Check sheet for the modelled part. Datum: model origin and axes. Units: mm. A direction names the side the tool comes from. Round coordinates to 2 decimals unless told otherwise and drop trailing zeros. Order: outer loops, then holes, each group sorted by start corner. A loop starts at its lowest first (then second) coordinate and runs counter-clockwise, first axis right, second up. Notation, with made-up numbers: (-38.75, 50) -> (-3.75, 50) arc R24 cw to (-3.75, 89) -> close; hole circle Ø2 at (27.5, 30.5). An arc over 180 degrees is marked (long way). Answer in a Markdown table with one row per item. Add a question column.
1. Depth check by flat-ended pin: P1, Ø10, axis at y = 105, z = 904.5, coming from the +X side; P2, Ø3, axis at x = 2, z = 1144.5, coming from the +Y side; P3, Ø1, axis at x = -12, z = 764.5, coming from the -Y side. Enter the tip coordinate at first touch or a pass-through.
2. Draft check along Z on faces 1 (the flat face through (9.3, 93.7, 1424)), 2 (the flat face through (0, 103, 1451)), 3 (the cylindrical face through (-1.82, 116.88, 1437.31)). Enter one of: +Z half, -Z half, draft (parallel to the pull), parting line (faces both ways), or undercut.
3. Material ranges on L1, parallel to Y at x = 5.5, z = -21.5; L2, parallel to Z at x = -13, y = 108.5; L3, parallel to Y at x = -2.5, z = 326.5, recorded low to high. Write a range as from..to.
4. Sectioned sample at C-C, the plane z = 386. Record the boundary of the cut face in (x, y).
5. Sectioned sample at A-A, the plane y = 103. Record the boundary of the cut face in (x, z), then the cut area to 3 significant figures.
6. Sectioned sample at B-B, the plane x = 0. Record the boundary of the cut face in (y, z), then the cut area to 3 significant figures.
7. Access from +Z, -Z, +X, -X, +Y, -Y to the whole of each face (thin tool, end or side, straight path). Record for faces 4 (the flat face through (-0.1, 116.4, 77)), 5 (the flat face through (0, 103, -127)).
```python
from build123d import *

# Parameters (mm, degrees)
CYLINDER031_R     = 15
CYLINDER031_DEPTH = 204
CYLINDER032_R     = 14
CYLINDER032_DEPTH = 27
CYLINDER030_R     = 13
CYLINDER030_DEPTH = 1390


with BuildPart() as obj1:
    # Cylinder031 → Cylinder031 (new body)
    with BuildSketch(Plane.XY):
        Circle(CYLINDER031_R)
    extrude(amount=CYLINDER031_DEPTH)


with BuildPart() as obj2:
    # Cylinder032 → Cylinder032 (new body)
    with BuildSketch(Plane.XY.offset(1363)):
        Circle(CYLINDER032_R)
    extrude(amount=CYLINDER032_DEPTH)


with BuildPart() as obj3:
    # Cylinder030 → Cylinder030 (new body)
    with BuildSketch(Plane.XY):
        Circle(CYLINDER030_R)
    extrude(amount=CYLINDER030_DEPTH)

    # Fusion006: union obj2
    add(obj2.part)


with BuildPart() as obj3_1:
    # Fusion006 placement: moved
    add(obj3.part.moved(Location((0, 0, 188))))

    # Fusion007: union obj1
    add(obj1.part)


with BuildPart() as obj3_2:
    # Fusion007 placement: moved
    add(obj3_1.part.moved(Location((0, 103, -127))))


solid = obj3_2.part
```
Answer key:
| question | item | result |
|---|---|---|
| 1 | P1 | stops at x = 13 |
| 1 | P2 | stops at y = 115.99 |
| 1 | P3 | stops at y = 96.94 |
| 2 | face 1 | undercut |
| 2 | face 2 | +Z half |
| 2 | face 3 | draft |
| 3 | L1 | y = 89.04..116.96 |
| 3 | L2 | z = -127..77 |
| 3 | L3 | y = 90.24..115.76 |
| 4 | outline | circle Ø26 at (0, 103) |
| 5 | outline | (-15, -127) -> (15, -127) -> (15, 77) -> (13, 77) -> (13, 1424) -> (14, 1424) -> (14, 1451) -> (-14, 1451) -> (-14, 1424) -> (-13, 1424) -> (-13, 77) -> (-15, 77) -> close |
| 5 | area | 41,900 mm² |
| 6 | outline | (88, -127) -> (118, -127) -> (118, 77) -> (116, 77) -> (116, 1424) -> (117, 1424) -> (117, 1451) -> (89, 1451) -> (89, 1424) -> (90, 1424) -> (90, 77) -> (88, 77) -> close |
| 6 | area | 41,900 mm² |
| 7 | face 4 | none |
| 7 | face 5 | -Z, +X, -X, +Y, -Y |
